Could you check a few things on this drawing? It's one solid part, dimensions in mm from its lowest x, y, z. Round coordinates to 2 decimals unless told otherwise and drop trailing zeros. Order: outer loops, then holes, each group sorted by start corner. A loop starts at its lowest first (then second) coordinate and runs counter-clockwise, first axis right, second up.
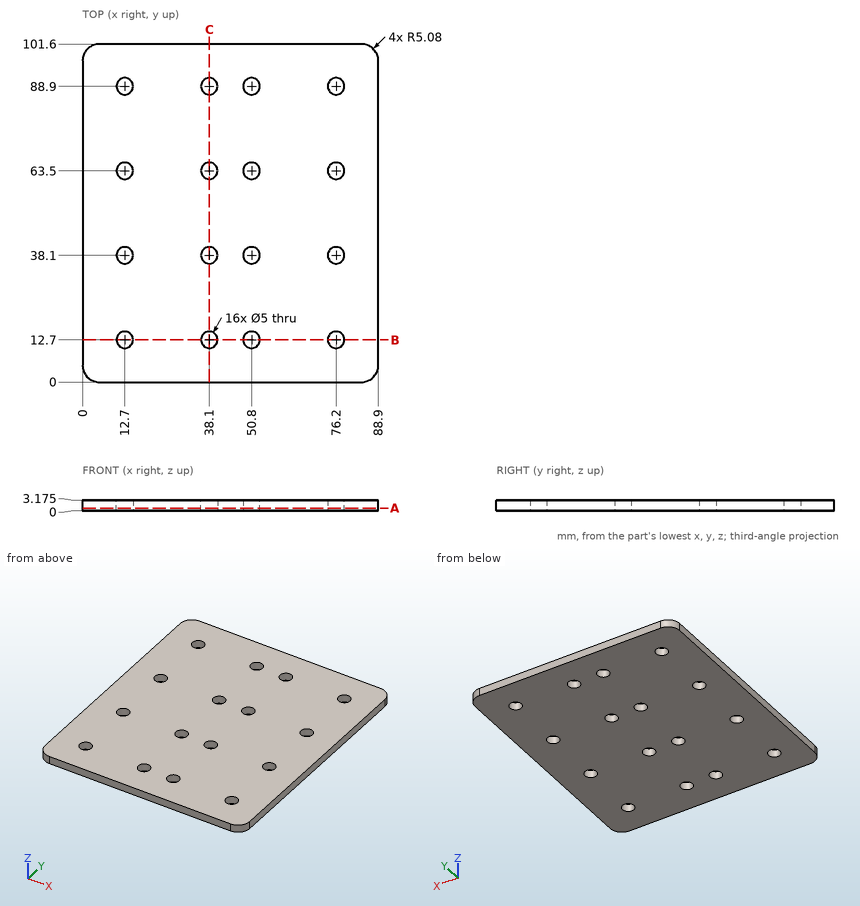
1) I'm going to push a flat-ended pin straight in: pin 1 (3 mm diameter, centred on x = 76.2, y = 38.1, fed in from -Z). Where does the tip first touch, or does it pass through?
2) If we section it at A-A (z = 0.8): Give the number of separate pieces and of enclosed holes in the cut face, plus the area to 3 significant figures.
3) I need wall thicknesses on line 1 (Y direction, x = 76.2, z = 0.9); line 2 (X direction, y = 40, z = 0.45); line 3 (X direction, y = 91, z = 2.1). Which ranges of each line are inside material? Lowest first, please.
4) If we section it at B-B (y = 12.7): Write out the boundary of the cut face in (x, z) (3 decimals), plus the area to 3 significant figures.
5) If we section it at C-C (x = 38.1): Write out the boundary of the cut face in (y, z) (3 decimals).
Solutions:
1. pin 1: passes through
2. separate pieces: 1
2. enclosed holes: 16
2. area: 8,700 mm2
3. line 1: y = 0 to 10.2, 15.2 to 35.6, 40.6 to 61, 66 to 86.4, 91.4 to 101.6
3. line 2: x = 0 to 11.08, 14.32 to 36.48, 39.72 to 49.18, 52.42 to 74.58, 77.82 to 88.9
3. line 3: x = 0 to 11.34, 14.06 to 36.74, 39.46 to 49.44, 52.16 to 74.84, 77.56 to 88.9
4. outline: (0, 0) - (10.2, 0) - (10.2, 3.175) - (0, 3.175) - close; (15.2, 0) - (35.6, 0) - (35.6, 3.175) - (15.2, 3.175) - close; (40.6, 0) - (48.3, 0) - (48.3, 3.175) - (40.6, 3.175) - close; (53.3, 0) - (73.7, 0) - (73.7, 3.175) - (53.3, 3.175) - close; (78.7, 0) - (88.9, 0) - (88.9, 3.175) - (78.7, 3.175) - close
4. area: 219 mm2
5. outline: (0, 0) - (10.2, 0) - (10.2, 3.175) - (0, 3.175) - close; (15.2, 0) - (35.6, 0) - (35.6, 3.175) - (15.2, 3.175) - close; (40.6, 0) - (61, 0) - (61, 3.175) - (40.6, 3.175) - close; (66, 0) - (86.4, 0) - (86.4, 3.175) - (66, 3.175) - close; (91.4, 0) - (101.6, 0) - (101.6, 3.175) - (91.4, 3.175) - close
